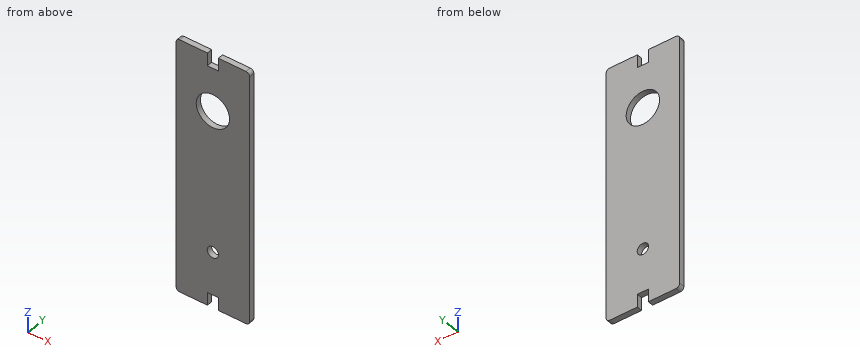
```python
from build123d import *

# Parameters (mm, degrees)
F1_DEPTH = 3
F4_D     = 18.15
F6_D     = 6.15
F7_R     = 2


with BuildPart() as f1:
    # F0 (on Front) → F1 (new body)
    with BuildSketch(Plane.XZ):
        Polygon((0, -124.5), (0, 0), (-3, 0), (-3, 7), (-20, 7), (-20, -131.5), (-3, -131.5), (-3, -124.5), align=None)
    extrude(amount=F1_DEPTH)

    # F2: F1 across plane


with BuildPart() as f1_1:
    add(f1.part)
    add(f1.part.mirror(Plane.YZ))

    # F4 (through all)
    with Locations(Plane.XZ.offset(3)):
        with Locations((0, -23.5)):
            Hole(F4_D / 2)

    # F6 (through all)
    with Locations(Plane.XZ.offset(3)):
        with Locations((0, -101)):
            Hole(F6_D / 2)

    # F7
    f7_edges = [f1_1.edges().sort_by_distance(p)[0] for p in [
        (20, -1.5, -131.5),
        (-20, -1.5, -131.5),
        (-20, -1.5, 7),
        (20, -1.5, 7),
    ]]
    fillet(f7_edges, radius=F7_R)


solid = f1_1.part
```
Could you check a few things on this model? Use its own coordinates, in mm. Coordinates: 2 decimals unless noted, no trailing zeros. Loops run counter-clockwise (first coordinate to the right, second up) from the corner with the lowest first, then second, coordinate; pieces in that order, holes last. Notation, with made-up numbers: M 40,31 L 51,31 A18 ccw 51,62 Z; hole C 56,15 d6. An arc over 180 degrees is marked long. Put each result on its own line as item: value. Start each with the question number.
(1) Suppose I cut it at D-D on x = -7. Please give me the cut outline in (y, z), then the cut area to 3 significant figures.
(2) Suppose I cut it at C-C on z = -101. Please give me the cut outline in (x, y) (3 decimals).
(3) Will these pins go through, and if not, where does the flat tip stop? P1, Ø1.5, axis at x = 1, y = -1, coming from the +Z side; P2, Ø5.5, axis at x = 0, z = -101, coming from the -Y side.
(4) Suppose I cut it at A-A on y = -0.85. Please give me the cut outline in (x, z) (3 decimals).
(5) I need wall thicknesses on line 1 (Z direction, x = 0, y = -1.7) (3 decimals); line 2 (Z direction, x = 0.5, y = -2.65); line 3 (X direction, y = -1.7, z = -26). Which ranges of each line are inside material? Lowest first, please. Write a range as from..to.
(6) Suppose I cut it at B-B on x = 0. Please give me the cut outline in (y, z) (3 decimals), then the cut area to 3 significant figures.
Solutions:
1. outline: M -3,-131.5 L 0,-131.5 L 0,-29.28 L -3,-29.28 Z; M -3,-17.72 L 0,-17.72 L 0,7 L -3,7 Z
1. area: 381 mm2
2. outline: M -20,-3 L -3.075,-3 L -3.075,0 L -20,0 Z; M 3.075,-3 L 20,-3 L 20,0 L 3.075,0 Z
3. P1: stops at z = 0
3. P2: passes through
4. outline: M -20,-129.5 A2 ccw -18,-131.5 L -3,-131.5 L -3,-124.5 L 3,-124.5 L 3,-131.5 L 18,-131.5 A2 ccw 20,-129.5 L 20,5 A2 ccw 18,7 L 3,7 L 3,0 L -3,0 L -3,7 L -18,7 A2 ccw -20,5 Z; hole C 0,-23.5 d18.15; hole C 0,-101 d6.15
5. line 1: z = -124.5..-104.075, -97.925..-32.575, -14.425..0
5. line 2: z = -124.5..-104.03, -97.97..-32.56, -14.44..0
5. line 3: x = -20..-8.72, 8.72..20
6. outline: M -3,-124.5 L 0,-124.5 L 0,-104.075 L -3,-104.075 Z; M -3,-97.925 L 0,-97.925 L 0,-32.575 L -3,-32.575 Z; M -3,-14.425 L 0,-14.425 L 0,0 L -3,0 Z
6. area: 301 mm2
